from build123d import *

# Parameters (mm, degrees)
F0_R     = 5
F1_DEPTH = 15


with BuildPart() as f1:
    # F0 (on Top) → F1 (new body)
    with BuildSketch(Plane.XY):
        with BuildLine():
            ThreePointArc((-73.026882, 17.090189), (-15.34069, 73.414326), (60.072808, 44.902758))
            Line((60.072808, 44.902758), (62.89309, 46.135228))
            Line((62.89309, 46.135228), (37.842179, 103.459659))
            ThreePointArc((37.842179, 103.459659), (29.246367, 111.198365), (17.761595, 109.82886))
            ThreePointArc((17.761595, 109.82886), (-19.853627, 95.011416), (-60.254823, 93.526516))
            ThreePointArc((-60.254823, 93.526516), (-71.327003, 90.18251), (-76.104701, 79.64927))
            Line((-76.104701, 79.64927), (-76.104701, 17.090189))
            Line((-76.104701, 17.090189), (-73.026882, 17.090189))
        make_face()
        with Locations((-62.104701, 79.64927)):
            Circle(F0_R, mode=Mode.SUBTRACT)
        with Locations((25.013633, 97.853555)):
            Circle(F0_R, mode=Mode.SUBTRACT)
    extrude(amount=F1_DEPTH)


solid = f1.part
The listing builds one solid part. Answer for the finished solid, in the listing's coordinates (mm). Give positions to 0.01 mm unless a question says otherwise; leave off trailing zeros. Loops run counter-clockwise (first coordinate to the right, second up) from the corner with the lowest first, then second, coordinate; pieces in that order, holes last.
Item 1: Each of these flat-tipped pins is pushed along its axis until it touches: pin 1 Ø6 at (x, y) = (-62.1, 79.65) entering from -Z; pin 2 Ø4 at (x, z) = (-14.5, 3.5) entering from +Y; pin 3 Ø4 at (x, z) = (32.5, 5.5) entering from -Y; pin 4 Ø6 at (x, z) = (-62, 2.5) entering from -Y. Where does it stop, or does it pass through?
Derived:
pin 1: passes through
pin 2: stops at y = 96.79
pin 3: stops at y = 66.59
pin 4: stops at y = 37.42
Item 2: A cutting plane is placed at A-A (y = 65). Give the vertices of the cut face in (x, z).
Derived:
outline: (-76.1, 0) - (-37.42, 0) - (-37.42, 15) - (-76.1, 15) - close; (37.42, 0) - (54.65, 0) - (54.65, 15) - (37.42, 15) - close
Item 3: Find the intervals of material crossed by line 1 along X through (y, z) = (58, 13); line 2 along X through (y, z) = (56, 3); line 3 along Y through (x, z) = (25, 1.75), in increasing order.
Derived:
line 1: x = -76.1 to -47.55, 47.55 to 57.71
line 2: x = -76.1 to -49.89, 49.89 to 58.58
line 3: y = 70.71 to 92.85, 102.85 to 111.85
Item 4: Determine the mould class of faces 1 (the flat face through (-76.105, 49, 7)), 2 (the cylindrical face through (-16.51, 73.16, 7.4)), 3 (the flat face through (-23, 76, 0)) for opening direction X: +X half, -X half, draft (parallel to the pull), parting line (faces both ways), or undercut.
Derived:
face 1: -X half
face 2: undercut
face 3: draft
Item 5: A cutting plane is placed at C-C (y = 35). Give the vertices of the cut face in (x, z), then the cut area to 3 significant figures.
Derived:
outline: (-76.1, 0) - (-66.33, 0) - (-66.33, 15) - (-76.1, 15) - close
area: 147 mm2
Item 6: A cutting plane is placed at D-D (x = -11.5). Give the vertices of the cut face in (y, z).
Derived:
outline: (74.11, 0) - (97.07, 0) - (97.07, 15) - (74.11, 15) - close
Item 7: A cutting plane is placed at B-B (z = 6). Give the vertices of the cut face in (x, y).
Derived:
outline: (-76.1, 17.09) - (-73.03, 17.09) arc R75 cw to (60.07, 44.9) - (62.89, 46.14) - (37.84, 103.46) arc R14 ccw to (17.76, 109.83) arc R120 cw to (-60.25, 93.53) arc R14 ccw to (-76.1, 79.65) - close; hole circle Ø10 at (-62.1, 79.65); hole circle Ø10 at (25.01, 97.85)
